Geometry check sheet. Reference: the model listing, model coordinates, mm. Face numbers are marked on the shaded views. Give positions to 0.01 mm unless a question says otherwise; leave off trailing zeros. Write each loop counter-clockwise with the first axis right and the second up, starting at its lowest first coordinate (ties: lowest second). Pieces come first, ordered by that corner, then holes.
(1) Mould release check, pull along Y, two halves, no side actions. Record for the marked faces 1, 2, 3 and 4: +Y half, -Y half, draft (parallel to the pull), parting line (faces both ways), or undercut.
(2) Cross-section at C-C (y = 838). Record the boundary of the cut face in (x, z), and give its area (3 significant figures).
(3) Cross-section at A-A (z = 15). Record the boundary of the cut face in (x, y).
(4) Cross-section at B-B (x = 71.5). Record the boundary of the cut face in (y, z).
(5) Depth check by flat-ended pin: P1, Ø6, axis at x = 159.89, y = 405.11, coming from the +Z side (3 decimals); P2, Ø8.5, axis at x = -12.11, y = -7.49, coming from the +Z side; P3, Ø6, axis at x = 64.5, z = 80, coming from the +Y side; P4, Ø2, axis at y = 307.5, z = 158.5, coming from the -X side. Enter the tip coordinate at first touch or a pass-through.
(6) Cross-section at D-D (z = 205). Record the boundary of the cut face in (x, y), and give its area (3 significant figures).
(7) Thickness scan on line 1 along Y through (x, z) = (69.5, 133.5); line 2 along X through (y, z) = (261, 84); line 3 along Z through (x, y) = (143, 668). Record the ranges inside material, lowest first.
```python
from build123d import *

# Parameters (mm, degrees)
F0_R     = 3.25
F1_DEPTH = 2
F3_DEPTH = 226
F5_DEPTH = 2
F7_DEPTH = 1220.99755
F8_R     = 5.25
F8_R_2   = 11.25
F8_R_3   = 4.25
F9_DEPTH = 25


with BuildPart() as f1:
    # F0 (on Top) → F1 (new body)
    with BuildSketch(Plane.XY):
        Polygon((-19.607349, 959.007126), (-19.607349, 942.007126), (150.392651, 942.007126), (150.392651, 2.007126), (-19.607349, 2.007126), (-19.607349, -14.992874), (167.392651, -14.992874), (167.392651, 959.007126), align=None)
        with Locations((-12.107349, -7.492874)):
            Circle(F0_R, mode=Mode.SUBTRACT)
        with Locations((159.892651, -7.492874)):
            Circle(F0_R, mode=Mode.SUBTRACT)
        with Locations((159.892651, 131.907126)):
            Circle(F0_R, mode=Mode.SUBTRACT)
        with Locations((159.892651, 268.507126)):
            Circle(F0_R, mode=Mode.SUBTRACT)
        with Locations((159.892651, 405.107126)):
            Circle(F0_R, mode=Mode.SUBTRACT)
        with Locations((-12.107349, 951.507126)):
            Circle(F0_R, mode=Mode.SUBTRACT)
        with Locations((159.892651, 541.707126)):
            Circle(F0_R, mode=Mode.SUBTRACT)
        with Locations((159.892651, 678.307126)):
            Circle(F0_R, mode=Mode.SUBTRACT)
        with Locations((159.892651, 814.907126)):
            Circle(F0_R, mode=Mode.SUBTRACT)
        with Locations((159.892651, 951.507126)):
            Circle(F0_R, mode=Mode.SUBTRACT)
    extrude(amount=F1_DEPTH)

    # F2 (on face) → F3 (join)
    with BuildSketch(Plane.XY.offset(2)):
        Polygon((-19.607349, 944.007126), (-19.607349, 942.007126), (150.392651, 942.007126), (150.392651, 2.007126), (-19.607349, 2.007126), (-19.607349, 0.007126), (152.392651, 0.007126), (152.392651, 944.007126), align=None)
    extrude(amount=F3_DEPTH)

    # F4 (on face) → F5 (join)
    with BuildSketch(Plane.XY.offset(228)):
        Polygon((152.392651, 944.007126), (-19.607349, 944.007126), (-19.607349, 927.007126), (135.392651, 927.007126), (135.392651, 17.007126), (-19.607349, 17.007126), (-19.607349, 0.007126), (152.392651, 0.007126), align=None)
    extrude(amount=F5_DEPTH)

    # F6 (on face) → F7 (cut)
    with BuildSketch(Plane(origin=(0, 959.007126, 0), x_dir=(-1, 0, 0), z_dir=(0, 1, 0))):
        with BuildLine():
            Line((-10.392651, 50), (-122.392651, 50))
            ThreePointArc((-122.392651, 50), (-125.928185, 48.535534), (-127.392651, 45))
            Line((-127.392651, 45), (-127.392651, -20.446198))
            Line((-127.392651, -20.446198), (-5.392651, -20.446198))
            Line((-5.392651, -20.446198), (-5.392651, 45))
            ThreePointArc((-5.392651, 45), (-6.857117, 48.535534), (-10.392651, 50))
        make_face()
    extrude(amount=-F7_DEPTH, mode=Mode.SUBTRACT)

    # F8 (on face) → F9 (cut)
    with BuildSketch(Plane.YZ.offset(152.392651)):
        with Locations((620.007126, 140)):
            Circle(F8_R)
        with Locations((650.007126, 140)):
            Circle(F8_R)
        with Locations((445.007126, 60)):
            Circle(F8_R_2)
        with Locations((415.007126, 60)):
            Circle(F8_R_3)
    extrude(amount=-F9_DEPTH, mode=Mode.SUBTRACT)


solid = f1.part
```
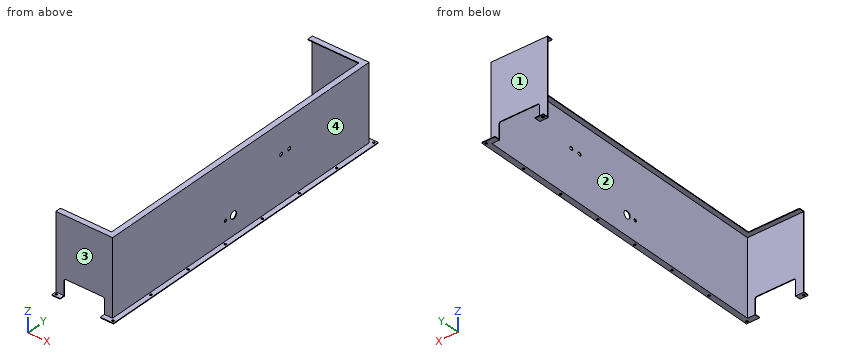
Reply:
1. face 1: +Y half
1. face 2: undercut
1. face 3: -Y half
1. face 4: draft
2. outline: (135.39, 228) - (150.39, 228) - (150.39, 0) - (167.39, 0) - (167.39, 2) - (152.39, 2) - (152.39, 230) - (135.39, 230) - close
2. area: 520 mm2
3. outline: (-19.61, 0.01) - (5.39, 0.01) - (5.39, 2.01) - (-19.61, 2.01) - close; (-19.61, 942.01) - (5.39, 942.01) - (5.39, 944.01) - (-19.61, 944.01) - close; (127.39, 0.01) - (152.39, 0.01) - (152.39, 944.01) - (127.39, 944.01) - (127.39, 942.01) - (150.39, 942.01) - (150.39, 2.01) - (127.39, 2.01) - close
4. outline: (0.01, 50) - (2.01, 50) - (2.01, 228) - (17.01, 228) - (17.01, 230) - (0.01, 230) - close; (927.01, 228) - (942.01, 228) - (942.01, 50) - (944.01, 50) - (944.01, 230) - (927.01, 230) - close
5. P1: passes through
5. P2: stops at z = 2
5. P3: stops at y = 944.01
5. P4: stops at x = 150.39
6. outline: (-19.61, 0.01) - (152.39, 0.01) - (152.39, 944.01) - (-19.61, 944.01) - (-19.61, 942.01) - (150.39, 942.01) - (150.39, 2.01) - (-19.61, 2.01) - close
6. area: 2,570 mm2
7. line 1: y = 0.01 to 2.01, 942.01 to 944.01
7. line 2: x = 150.39 to 152.39
7. line 3: z = 228 to 230
